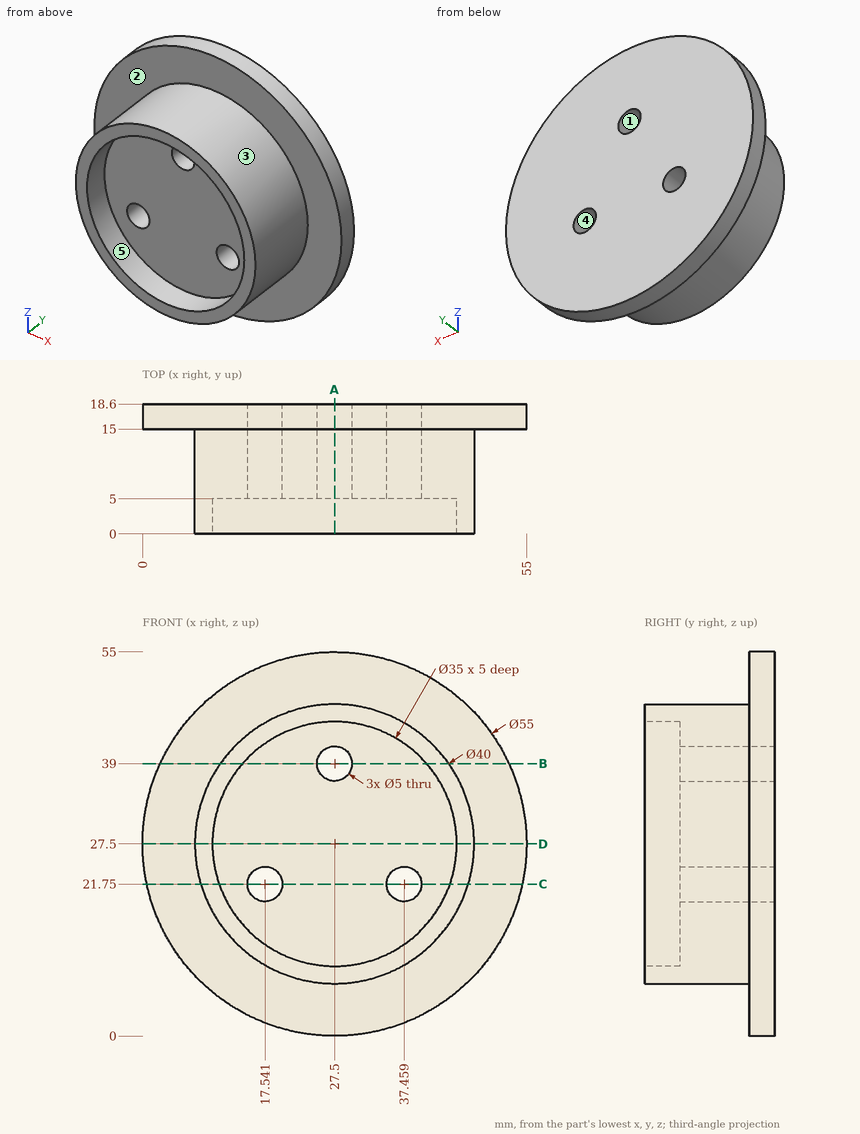
The figure shows three views and two pictorial views of one solid part (mm, origin at its lowest corner). Answer the questions. A direction names the side the tool comes from. Give positions to 0.01 mm unless a question says otherwise; leave off trailing zeros. Loops run counter-clockwise (first coordinate to the right, second up) from the corner with the lowest first, then second, coordinate; pieces in that order, holes last. Notation, with made-up numbers: (73, -33.75) -> (131, -33.75) arc R20 ccw to (131, 0.25) -> close; hole circle Ø4 at (49, -30.5). An arc over 180 degrees is marked (long way). Use a Markdown table: item, result. Add a question column.
1. Section C-C on z = 21.75 is taken. Determine the outline of the cut face in (x, y).
2. Section A-A on x = 27.5 is taken. Determine the outline of the cut face in (y, z).
3. Determine the mould class of the marked faces 1, 2 and 3 for opening direction X: released by +X, released by -X, zero draft, split by the parting line, or undercut.
4. Flat-ended cylindrical pins translate along their axes: pin 1 Ø1 at (x, z) = (32, 38.5) entering from -Y; pin 2 Ø5 at (y, z) = (11.5, 8.5) entering from -X; pin 3 Ø2 at (x, y) = (23.5, 11) entering from +Z. Find the tip coordinate at first contact, or state that the pin passes through.
5. Section D-D on z = 27.5 is taken. Determine the outline of the cut face in (x, y), and give its area (3 significant figures).
6. For the marked faces 4 and 5, determine the directions among +Z, -Z, +X, -X, +Y, -Y from which every point of the face is accessible in a straight line to the end or side of a thin tool.
7. Find the intervals of material crossed by probe 1 along X at (y, z) = (15.25, 21.75); probe 2 along X at (y, z) = (13.25, 21.75) (1 decimal); probe 3 along Z at (x, y) = (27.5, 2.15), in increasing order.
8. Section B-B on z = 39 is taken. Determine the outline of the cut face in (x, y).
Results below:
| question | item | result |
|---|---|---|
| 1 | outline | (0.61, 15) -> (8.34, 15) -> (8.34, 0) -> (10.97, 0) -> (10.97, 5) -> (15.04, 5) -> (15.04, 18.6) -> (0.61, 18.6) -> close; (20.04, 5) -> (34.96, 5) -> (34.96, 18.6) -> (20.04, 18.6) -> close; (39.96, 5) -> (44.03, 5) -> (44.03, 0) -> (46.66, 0) -> (46.66, 15) -> (54.39, 15) -> (54.39, 18.6) -> (39.96, 18.6) -> close |
| 2 | outline | (0, 7.5) -> (15, 7.5) -> (15, 0) -> (18.6, 0) -> (18.6, 36.5) -> (5, 36.5) -> (5, 10) -> (0, 10) -> close; (0, 45) -> (5, 45) -> (5, 41.5) -> (18.6, 41.5) -> (18.6, 55) -> (15, 55) -> (15, 47.5) -> (0, 47.5) -> close |
| 3 | face 1 | undercut |
| 3 | face 2 | zero draft |
| 3 | face 3 | split by the parting line |
| 4 | pin 1 | stops at y = 5 |
| 4 | pin 2 | stops at x = 16.2 |
| 4 | pin 3 | stops at z = 47.27 |
| 5 | outline | (0, 15) -> (7.5, 15) -> (7.5, 0) -> (10, 0) -> (10, 5) -> (45, 5) -> (45, 0) -> (47.5, 0) -> (47.5, 15) -> (55, 15) -> (55, 18.6) -> (0, 18.6) -> close |
| 5 | area | 623 mm^2 |
| 6 | face 4 | +Y, -Y |
| 6 | face 5 | -Y |
| 7 | probe 1 | x = 0.61 to 15.04, 20.04 to 34.96, 39.96 to 54.39 |
| 7 | probe 2 | x = 8.3 to 15, 20 to 35, 40 to 46.7 |
| 7 | probe 3 | z = 7.5 to 10, 45 to 47.5 |
| 8 | outline | (2.52, 15) -> (11.14, 15) -> (11.14, 0) -> (14.31, 0) -> (14.31, 5) -> (25, 5) -> (25, 18.6) -> (2.52, 18.6) -> close; (30, 5) -> (40.69, 5) -> (40.69, 0) -> (43.86, 0) -> (43.86, 15) -> (52.48, 15) -> (52.48, 18.6) -> (30, 18.6) -> close |
